from build123d import *

# Parameters (mm, degrees)
SKETCH1_R           = 50.8
BOSS_EXTRUDE1_DEPTH = 254
SKETCH2_W           = 63.5
SKETCH2_H           = 79.31147458
BOSS_EXTRUDE2_DEPTH = 46.99
SKETCH3_W           = 25.4
SKETCH3_H           = 79.31147458
CUT_EXTRUDE1_DEPTH  = 63.5
FILLET1_R           = 25.4
SKETCH7_W           = 25.4
SKETCH7_H           = 98.373776994
BOSS_EXTRUDE3_DEPTH = 63.5
SKETCH8_R           = 12.7
CUT_EXTRUDE5_DEPTH  = 312.781766786
FILLET2_R           = 25.4
SKETCH6_R           = 12.7
BOSS_EXTRUDE4_DEPTH = 53.34


with BuildPart() as part:
    # Sketch1 → Boss-Extrude1 (new body)
    with BuildSketch(Plane(origin=(0, 0, 0), x_dir=(1, 0, 0), z_dir=(0, 1, 0))):
        with Locations(Location((0, 0, 0), (0, 0, 270))):
            Circle(SKETCH1_R)
    extrude(amount=BOSS_EXTRUDE1_DEPTH)

    # Sketch2 → Boss-Extrude2 (add)
    with BuildSketch(Plane(origin=(0, 254, 0), x_dir=(1, 0, 0), z_dir=(0, 1, 0))):
        Rectangle(SKETCH2_W, SKETCH2_H)
    extrude(amount=BOSS_EXTRUDE2_DEPTH)

    # Sketch3 → Cut-Extrude1 (cut)
    with BuildSketch(Plane(origin=(0, 300.99, 0), x_dir=(1, 0, 0), z_dir=(0, 1, 0))):
        Rectangle(SKETCH3_W, SKETCH3_H)
    extrude(amount=-CUT_EXTRUDE1_DEPTH, mode=Mode.SUBTRACT)

    # Fillet1
    fillet1_edges = [part.edges().sort_by_distance(p)[0] for p in [
        (22.225, 300.99, -39.65573729),
        (-22.225, 300.99, 39.65573729),
        (-22.225, 300.99, -39.65573729),
        (22.225, 300.99, 39.65573729),
    ]]
    fillet(fillet1_edges, radius=FILLET1_R)

    # Sketch7 → Boss-Extrude3 (add)
    with BuildSketch(Plane.XZ):
        Rectangle(SKETCH7_W, SKETCH7_H)
    extrude(amount=BOSS_EXTRUDE3_DEPTH)

    # Sketch8 → Cut-Extrude5 (cut, through all)
    with BuildSketch(Plane(origin=(12.7, 0, 0), x_dir=(0, 0, -1), z_dir=(1, 0, 0))):
        with Locations((0, -31.75)):
            Circle(SKETCH8_R)
    extrude(amount=-CUT_EXTRUDE5_DEPTH, mode=Mode.SUBTRACT)

    # Fillet2
    fillet2_edges = [part.edges().sort_by_distance(p)[0] for p in [
        (0, -63.5, 49.186888497),
        (0, -63.5, -49.186888497),
    ]]
    fillet(fillet2_edges, radius=FILLET2_R)

    # Sketch6 → Boss-Extrude4 (add)
    with BuildSketch(Plane(origin=(31.75, 0, 0), x_dir=(0, 0, -1), z_dir=(1, 0, 0))):
        with Locations((0, 286.494432144)):
            Circle(SKETCH6_R)
    extrude(amount=-BOSS_EXTRUDE4_DEPTH)


solid = part.part
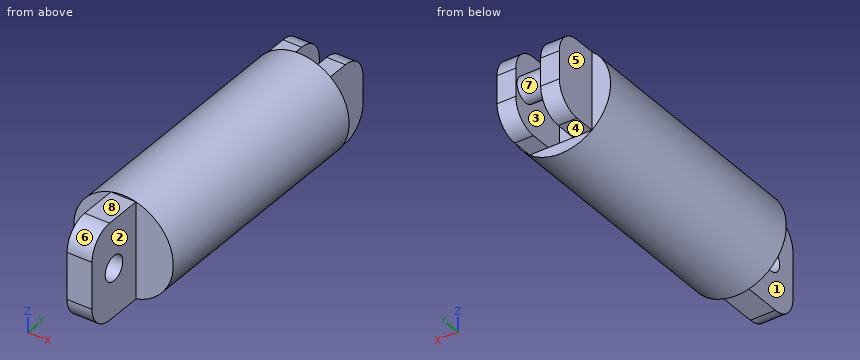
Design review of the part built by this model. Coordinates are the model's own, in mm. Face numbers are marked on the shaded views. A direction names the side the tool comes from. Round coordinates to 2 decimals unless told otherwise and drop trailing zeros. Write each loop counter-clockwise with the first axis right and the second up, starting at its lowest first coordinate (ties: lowest second). Pieces come first, ordered by that corner, then holes. Notation, with made-up numbers: M -24,84.5 L 25,84.5 A33 cw 25,119.5 Z; hole C 52.25,8 d7. An arc over 180 degrees is marked long. One line per item, written item: value. Start each with the question number.
1. Take a section at D-D on z = -35. State the section outline as (x, y) points.
2. Clearance check with flat-ended pins moving along their axes: P1, Ø10, axis at y = 110.5, z = 36.5, coming from the -X side; P2, Ø12.5, axis at x = -8, z = -46.5, coming from the +Y side; P3, Ø19, axis at y = -18, z = -2.5, coming from the +X side; P4, Ø12, axis at x = 14, z = -7, coming from the -Y side. State where each tip first meets the part, or that it passes through.
3. Take a section at C-C on x = -4.5. State the section outline as (y, z) points.
4. Take a section at B-B on z = 0. State the section outline as (x, y) points, then the cut area to 3 significant figures.
5. To check wall thickness, follow probe 1 along Y at (x, z) = (6, 0); probe 2 along Z at (x, y) = (-1, -31); probe 3 along X at (y, z) = (270, -32). State the ranges of each line that lie inside material, in increasing order. Write a range as from..to.
6. For the marked faces 1, 2, 3, 4 and 5, list the 3-axis set-ups (+Z, -Z, +X, -X, +Y, -Y) from which the entire face can be reached by the end or side of a thin tool; tool diameter is ignored.
7. Draft analysis for pull direction Y (two halves, no side actions). For the marked faces 6, 7 and 8, state which applies: pulls with the +Y half, pulls with the -Y half, needs draft (parallel to the pull), parting line crosses it, or undercut.
8. Take a section at A-A on y = 268.5. State the section outline as (x, z) points, then the cut area to 3 significant figures.
Computed:
1. outline: M -36.82,0 L -12.7,0 L -12.7,-60.89 L 12.7,-60.89 L 12.7,0 L 36.82,0 L 36.82,254 L 31.75,254 L 31.75,290.25 L 12.7,290.25 L 12.7,237.49 L -12.7,237.49 L -12.7,290.25 L -31.75,290.25 L -31.75,254 L -36.82,254 Z
2. P1: stops at x = -39.85
2. P2: stops at y = 254
2. P3: stops at x = 12.7
2. P4: stops at y = -63.5
3. outline: M -63.5,-23.79 A25.4 ccw -38.1,-49.19 L 0,-49.19 L 0,-50.6 L 254,-50.6 L 254,-39.66 L 237.49,-39.66 L 237.49,39.66 L 254,39.66 L 254,50.6 L 0,50.6 L 0,49.19 L -38.1,49.19 A25.4 ccw -63.5,23.79 Z; C 286.49,0 d25.4; hole C -31.75,0 d25.4
4. outline: M -50.8,0 L -12.7,0 L -12.7,-19.05 L 12.7,-19.05 L 12.7,0 L 50.8,0 L 50.8,254 L 31.75,254 L 31.75,300.99 L 12.7,300.99 L 12.7,299.19 L -12.7,299.19 L -12.7,300.99 L -31.75,300.99 L -31.75,254 L -50.8,254 Z; M -12.7,-63.5 L 12.7,-63.5 L 12.7,-44.45 L -12.7,-44.45 Z; hole M -12.7,237.49 L 12.7,237.49 L 12.7,273.79 L -12.7,273.79 Z
4. area: 28,800 mm²
5. probe 1: y = -63.5..-44.45, -19.05..237.49, 273.79..299.19
5. probe 2: z = -49.19..-12.68, 12.68..49.19
5. probe 3: x = -31.75..-12.7, 12.7..31.75
6. face 1: +Z, -Z, -X, -Y
6. face 2: +Z, -Z, +X, -Y
6. face 3: none
6. face 4: -Z, +X, -X, +Y
6. face 5: +Z, -Z, -X, +Y
7. face 6: pulls with the -Y half
7. face 7: undercut
7. face 8: needs draft
8. outline: M -31.75,-39.66 L -12.7,-39.66 L -12.7,39.66 L -31.75,39.66 Z; M 12.7,-39.66 L 31.75,-39.66 L 31.75,39.66 L 12.7,39.66 Z
8. area: 3,020 mm²
